from build123d import *

# Parameters (mm, degrees)
SKETCH2_W               = 30
SKETCH2_H               = 8
SKETCH2_W_2             = 20
SKETCH2_H_2             = 5
BOSS_EXTRUDE1_DEPTH     = 30
SKETCH3_R               = 11
CUT_EXTRUDE1_DEPTH      = 55.626001135
FILLET1_R               = 10
FILLET2_R               = 0.5
SKETCH4_R               = 2
CUT_EXTRUDE2_DEPTH      = 61.018663764
SKETCH5_W               = 6
SKETCH5_H               = 2
CUT_EXTRUDE3_DEPTH      = 55.626001135
SKETCH6_W               = 14
SKETCH6_H               = 4
SKETCH6_W_2             = 12.707178849
BOSS_EXTRUDE2_DEPTH     = 8
CUT_EXTRUDE4_DEPTH      = 58.823956973
CUT_EXTRUDE4_DEPTH_BACK = 58.823956973
SKETCH7_R               = 1.5
SKETCH8_W               = 30
SKETCH8_H               = 25
SKETCH8_R               = 2
BOSS_EXTRUDE3_DEPTH     = 6
SKETCH9_R               = 2
BOSS_EXTRUDE4_DEPTH     = 4


with BuildPart() as part:
    # Sketch2 → Boss-Extrude1 (new body)
    with BuildSketch(Plane(origin=(0, 0, 0), x_dir=(0, 0, -1), z_dir=(1, 0, 0))):
        with Locations((25, -0.1)):
            Rectangle(SKETCH2_W, SKETCH2_H)
        Polygon((10, 15.1), (10, 10.1), (10, 3.9), (15, 3.9), (15, 15.1), align=None)
        with Locations((0, 12.6)):
            Rectangle(SKETCH2_W_2, SKETCH2_H_2)
        with Locations((0, -14.1)):
            Rectangle(SKETCH2_W_2, SKETCH2_H)
        Polygon((15, -4.1), (10, -4.1), (10, -10.1), (10, -18.1), (15, -18.1), align=None)
    extrude(amount=BOSS_EXTRUDE1_DEPTH)

    # Sketch3 → Cut-Extrude1 (cut, through all)
    with BuildSketch(Plane(origin=(0, 3.9, 0), x_dir=(1, 0, 0), z_dir=(0, 1, 0))):
        with Locations(Location((15, 26.775, 0), (0, 0, 270))):
            Circle(SKETCH3_R)
    extrude(amount=-CUT_EXTRUDE1_DEPTH, mode=Mode.SUBTRACT)

    # Fillet1
    fillet1_edges = [part.edges().sort_by_distance(p)[0] for p in [
        (0, -0.1, -40),
        (30, -0.1, -40),
    ]]
    fillet(fillet1_edges, radius=FILLET1_R)

    # Fillet2
    fillet2_edges = [part.edges().sort_by_distance(p)[0] for p in [
        (15, -10.1, -10),
        (15, 10.1, -10),
        (15, 15.1, -15),
        (15, 3.9, -15),
    ]]
    fillet(fillet2_edges, radius=FILLET2_R)

    # Sketch4 → Cut-Extrude2 (cut, through all)
    with BuildSketch(Plane(origin=(0, 15.1, 0), x_dir=(1, 0, 0), z_dir=(0, 1, 0))):
        with Locations(Location((7, 0, 0), (0, 0, 270))):
            Circle(SKETCH4_R)
        with Locations(Location((23, 0, 0), (0, 0, 270))):
            Circle(SKETCH4_R)
    extrude(amount=-CUT_EXTRUDE2_DEPTH, mode=Mode.SUBTRACT)

    # Sketch5 → Cut-Extrude3 (cut, through all)
    with BuildSketch(Plane(origin=(0, 3.9, 0), x_dir=(1, 0, 0), z_dir=(0, 1, 0))):
        with Locations((3, 31)):
            Rectangle(SKETCH5_W, SKETCH5_H)
    extrude(amount=-CUT_EXTRUDE3_DEPTH, mode=Mode.SUBTRACT)

    # Sketch6 → Boss-Extrude2 (add)
    with BuildSketch(Plane(origin=(0, 3.9, 0), x_dir=(1, 0, 0), z_dir=(0, 1, 0))):
        with Locations((-1.679843749, 34)):
            Rectangle(SKETCH6_W, SKETCH6_H)
        with Locations((-2.326254324, 28)):
            Rectangle(SKETCH6_W_2, SKETCH6_H)
    extrude(amount=-BOSS_EXTRUDE2_DEPTH)

    # Sketch7 → Cut-Extrude4 (cut, two sides: drawn at the far end of the back side and taken through both)
    with BuildSketch(Plane(origin=(0, 0, -36), x_dir=(-1, 0, 0), z_dir=(0, 0, -1)).offset(-CUT_EXTRUDE4_DEPTH_BACK)):
        with Locations(Location((4.679843749, -0.1, 0), (0, 0, 180))):
            Circle(SKETCH7_R)
    extrude(amount=CUT_EXTRUDE4_DEPTH + CUT_EXTRUDE4_DEPTH_BACK, mode=Mode.SUBTRACT)

    # Sketch8 → Boss-Extrude3 (add)
    with BuildSketch(Plane.XZ.offset(18.1)):
        with Locations((15, -2.5)):
            Rectangle(SKETCH8_W, SKETCH8_H)
        with Locations(Location((7, 0, 0), (0, 0, 90))):
            Circle(SKETCH8_R, mode=Mode.SUBTRACT)
        with Locations(Location((23, 0, 0), (0, 0, 90))):
            Circle(SKETCH8_R, mode=Mode.SUBTRACT)
    extrude(amount=BOSS_EXTRUDE3_DEPTH)

    # Sketch9 → Boss-Extrude4 (add)
    with BuildSketch(Plane.XZ.offset(24.1)):
        with BuildLine():
            Line((0, -30), (0, -15))
            Line((0, -15), (0, 10))
            Line((0, 10), (30, 10))
            Line((30, 10), (30, -15))
            Line((30, -15), (30, -30))
            ThreePointArc((30, -30), (27.071067812, -37.071067812), (20, -40))
            Line((20, -40), (10, -40))
            ThreePointArc((10, -40), (2.928932188, -37.071067812), (0, -30))
        make_face()
        with Locations(Location((7, 0, 0), (0, 0, 90))):
            Circle(SKETCH9_R, mode=Mode.SUBTRACT)
        with Locations(Location((23, 0, 0), (0, 0, 90))):
            Circle(SKETCH9_R, mode=Mode.SUBTRACT)
    extrude(amount=BOSS_EXTRUDE4_DEPTH)


solid = part.part
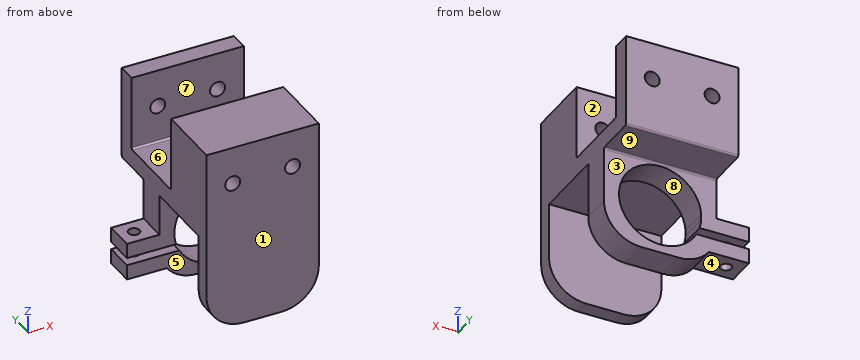
Geometry: final body of the model. Coordinates: model frame, mm. Face numbers are marked on the shaded views. A direction names the side the tool comes from. Give positions to 0.01 mm unless a question says otherwise; leave off trailing zeros. Write each loop counter-clockwise with the first axis right and the second up, starting at its lowest first coordinate (ties: lowest second). Pieces come first, ordered by that corner, then holes. Notation, with made-up numbers: (-18, -7) -> (6, -7) arc R16 cw to (6, 11) -> close; hole circle Ø2 at (65.25, -4.75). An arc over 180 degrees is marked (long way). Answer as a JSON object with one key per item and string values.
1. Mould query, pull axis Z, two halves, no side actions, for the marked faces 6, 7, 8 and 9. Classes: pulls with the +Z half, pulls with the -Z half, needs draft (parallel to the pull), parting line crosses it, or undercut.
Ans:
{"face 6": "pulls with the +Z half", "face 7": "needs draft", "face 8": "undercut", "face 9": "pulls with the -Z half"}
2. Access query for the marked faces 1, 2, 3, 4 and 5. Directions: +Z, -Z, +X, -X, +Y, -Y. A direction counts if a zero-diameter tool reaches every point of the face in a straight line with its end or side. Return the directions, or none.
Ans:
{"face 1": "+Z, -Z, +X, -X, -Y", "face 2": "+Z, +X, -X", "face 3": "-Z, +X, -X, +Y", "face 4": "-Z, -X, +Y, -Y", "face 5": "-Z, +X, -X"}
3. Cut plane C-C on z = -8.5. Output: boundary loops of the cut face in (x, y).
Ans:
{"outline": "(0, -28.1) -> (30, -28.1) -> (30, -10.1) -> (0, -10.1) -> close; (0, 10.1) -> (30, 10.1) -> (30, 15.1) -> (0, 15.1) -> close"}
4. Contact query for flat-ended pins moving along their axis: pin 1 (11 mm diameter, centred on x = 7.5, y = 11, fed in from -Z); pin 2 (17.5 mm diameter, centred on x = 15, z = -26.775, fed in from +Y); pin 3 (10 mm diameter, centred on x = 2, z = -22.5, fed in from +Y); pin 4 (10 mm diameter, centred on y = -18, z = -30, fed in from -X). Output: stop coordinate, or through.
Ans:
{"pin 1": "stops at z = -15", "pin 2": "stops at y = -24.1", "pin 3": "stops at y = 3.9", "pin 4": "passes through"}
5. Ray query, probe 1 along X at (y, z) = (-19, 0); probe 2 along Z at (x, y) = (15, 0.75) (3 decimals); probe 3 along Y at (x, z) = (8, -5.5). Return the intervals inside material, ascending. Write a range as from..to.
Ans:
{"probe 1": "x = 0..5, 9..21, 25..30", "probe 2": "z = -40..-37.775, -15.775..-10", "probe 3": "y = -28.1..-10.1, 10.1..15.1"}
6. Cut plane D-D on y = -0.1. Output: boundary loops of the cut face in (x, z) (3 decimals), and give its area (3 significant figures).
Ans:
{"outline": "(-8.68, -36) -> (-6.18, -36) -> (-6.18, -32) -> (-8.68, -32) -> close; (-8.68, -30) -> (-6.18, -30) -> (-6.18, -26) -> (-8.68, -26) -> close; (-3.18, -36) -> (2, -36) arc R10 ccw to (10, -40) -> (20, -40) arc R10 ccw to (30, -30) -> (30, -10) -> (0, -10) -> (0, -26) -> (-3.18, -26) -> (-3.18, -30) -> (4.483, -30) arc R11 cw to (4.027, -27.55) -> (4.027, -26) arc R11 cw (long way) to (5.32, -32) -> (-3.18, -32) -> close", "area": "517 mm^2"}
7. Cut plane A-A on z = 0. Output: boundary loops of the cut face in (x, y), and give its area (3 significant figures).
Ans:
{"outline": "(0, -28.1) -> (5, -28.1) -> (5, -10.1) -> (0, -10.1) -> close; (0, 10.1) -> (5, 10.1) -> (5, 15.1) -> (0, 15.1) -> close; (9, -28.1) -> (21, -28.1) -> (21, -10.1) -> (9, -10.1) -> close; (9, 10.1) -> (21, 10.1) -> (21, 15.1) -> (9, 15.1) -> close; (25, -28.1) -> (30, -28.1) -> (30, -10.1) -> (25, -10.1) -> close; (25, 10.1) -> (30, 10.1) -> (30, 15.1) -> (25, 15.1) -> close", "area": "506 mm^2"}
8. Cut plane B-B on x = 15. Output: boundary loops of the cut face in (y, z) (3 decimals), and give its area (3 significant figures).
Ans:
{"outline": "(-28.1, -40) -> (-24.1, -40) -> (-24.1, -15) -> (-4.1, -15) -> (-4.1, -15.775) -> (3.9, -15.775) -> (3.9, -15.5) arc R0.5 cw to (4.4, -15) -> (14.6, -15) arc R0.5 ccw to (15.1, -14.5) -> (15.1, 10) -> (10.1, 10) -> (10.1, -9.5) arc R0.5 cw to (9.6, -10) -> (-9.6, -10) arc R0.5 cw to (-10.1, -9.5) -> (-10.1, 10) -> (-28.1, 10) -> close; (-4.1, -40) -> (3.9, -40) -> (3.9, -37.775) -> (-4.1, -37.775) -> close", "area": "800 mm^2"}
